Geometry: final body of the model. Coordinates: model frame, mm. Face numbers are marked on the shaded views. A direction names the side the tool comes from. Coordinates: 2 decimals unless noted, no trailing zeros. Order: outer loops, then holes, each group sorted by start corner. A loop starts at its lowest first (then second) coordinate and runs counter-clockwise, first axis right, second up. Notation, with made-up numbers: (-36.5, -21.75) -> (17.5, -21.75) arc R10 cw to (17.5, -8.75) -> close; hole circle Ø10 at (83.25, -27). An arc over 180 degrees is marked (long way). Answer in a Markdown table with one row per item. Add a question column.
1) Section query B-B on y = 15. Return the cut outline in (x, z), then the cut area to 3 significant figures.
2) Section query A-A on z = 0. Count the separate pieces of the cut face and the enclosed holes in it, then the cut area to 3 significant figures.
3) Pull-direction query (Z, two-part tool) for the marked faces 1, 2 and 3; classes: +Z half, -Z half, draft (parallel to the pull), parting line (faces both ways), or undercut.
4) Ray query, line 1 (Y direction, x = 16, z = 0); line 2 (X direction, y = 29, z = 0); line 3 (Y direction, x = -1, z = -19). Return the intervals inside material, ascending. Write a range as from..to.
5) Section query D-D on z = 50. Return the cut outline in (x, y), then the cut area to 3 significant figures.
6) Set-up query: the marked faces 4 and 5. Return all of +Z, -Z, +X, -X, +Y, -Y with unobstructed straight access to the full face (end or side cutting, diameter ignored); none if empty.
7) Section query C-C on x = 50. Return the cut outline in (y, z).
8) Contact query for flat-ended pins moving along their axis: P1, Ø12, axis at x = -35, z = 47, coming from the -Y side; P2, Ø8, axis at y = 15, z = 0, coming from the -X side; P3, Ø2, axis at x = -50, z = -0.5, coming from the +Y side; P4, Ø3, axis at y = 15, z = 0, coming from the +X side. Output: stop coordinate, or through.
```python
from build123d import *

# Parameters (mm, degrees)
R_P_TITION_CIRCULAIRE1_COUNT = 4
ESQUISSE3_R                  = 2.5
ENL_V_MAT_EXTRU_1_DEPTH      = 22.5
CHANFREIN1_SIZE              = 1


with BuildPart() as part:
    # Esquisse1 → Base-Révolution (revolve)
    with BuildSketch(Plane.XY, mode=Mode.PRIVATE) as base_r_volution_sk:
        Polygon((9, 0), (22.5, 0), (22.5, 35), (59, 35), (59, 45), (20, 45), (20, 50), (9, 50), align=None)
    revolve(base_r_volution_sk.sketch.rotate(Axis((0, 0, 0), (0, 1, 0)), 90), axis=Axis((0, 0, 0), (0, 1, 0)))

    # Esquisse2 → Enlever de la matière-Révolution1 (revolve, cut)
    with BuildSketch(Plane.XY, mode=Mode.PRIVATE) as enlever_de_la_mati_re_r_volution1_sk:
        Polygon((50, 45), (45.5, 45), (47.809401077, 41), (50, 41), align=None)
    enlever_de_la_mati_re_r_volution1 = revolve(enlever_de_la_mati_re_r_volution1_sk.sketch.rotate(Axis((50, 50.797703058, 0), (0, -1, 0)), 270), axis=Axis((50, 50.797703058, 0), (0, -1, 0)), mode=Mode.SUBTRACT)

    # Répétition circulaire1: Enlever de la matière-Révolution1 ×4 about axis
    r_p_tition_circulaire1_axis = Axis((0, 0, 0), (0, 1, 0))
    for i in range(1, R_P_TITION_CIRCULAIRE1_COUNT):
        add(enlever_de_la_mati_re_r_volution1.rotate(r_p_tition_circulaire1_axis, i * 360 / R_P_TITION_CIRCULAIRE1_COUNT), mode=Mode.SUBTRACT)

    # Esquisse3 → Enlèv. mat.-Extru.1 (cut, symmetric)
    with BuildSketch(Plane(origin=(0, 0, 0), x_dir=(0, 0, -1), z_dir=(1, 0, 0))):
        with Locations((0, 15)):
            Circle(ESQUISSE3_R)
    extrude(amount=ENL_V_MAT_EXTRU_1_DEPTH, both=True, mode=Mode.SUBTRACT)

    # Chanfrein1
    chanfrein1_edges = [part.edges().sort_by_distance(p)[0] for p in [
        (0, 50, 20),
    ]]
    chamfer(chanfrein1_edges, length=CHANFREIN1_SIZE)


solid = part.part
```
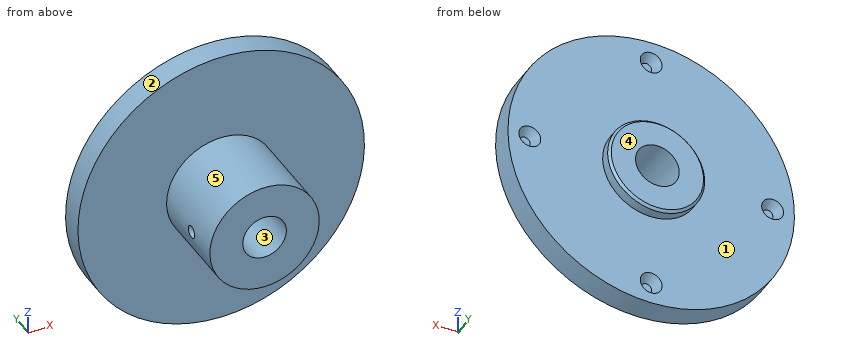
Result:
| question | item | result |
|---|---|---|
| 1 | outline | (-22.36, -2.5) arc R22.5 ccw to (22.36, -2.5) -> (8.65, -2.5) arc R9 cw to (-8.65, -2.5) -> close; (-22.36, 2.5) -> (-8.65, 2.5) arc R9 cw to (8.65, 2.5) -> (22.36, 2.5) arc R22.5 ccw to start |
| 1 | area | 1,200 mm2 |
| 2 | separate pieces | 4 |
| 2 | enclosed holes | 0 |
| 2 | area | 1,870 mm2 |
| 3 | face 1 | draft |
| 3 | face 2 | parting line |
| 3 | face 3 | undercut |
| 4 | line 1 | 0..12.5, 17.5..50 |
| 4 | line 2 | -22.5..-9, 9..22.5 |
| 4 | line 3 | 0..49.97 |
| 5 | outline | (-31.32, 35) -> (31.32, 35) -> (31.32, 45) -> (4.5, 45) -> (2.19, 41) -> (-2.19, 41) -> (-4.5, 45) -> (-31.32, 45) -> close |
| 5 | area | 600 mm2 |
| 6 | face 4 | +Z, -Z, +X, -X, +Y |
| 6 | face 5 | -Y |
| 7 | outline | (35, -31.32) -> (45, -31.32) -> (45, -4.5) -> (41, -2.19) -> (41, 2.19) -> (45, 4.5) -> (45, 31.32) -> (35, 31.32) -> close |
| 8 | P1 | y = 35 |
| 8 | P2 | x = -22.5 |
| 8 | P3 | y = 41 |
| 8 | P4 | through |
